Input: part model. Units: mm. Frame: model coordinates. Face numbers are marked on the shaded views. A direction names the side the tool comes from. Give positions to 0.01 mm unless a question says otherwise; leave off trailing zeros. Order: outer loops, then holes, each group sorted by start corner. A loop starts at its lowest first (then second) coordinate and runs counter-clockwise, first axis right, second up. Notation, with made-up numbers: (51, -10.75) - (102, -10.75) arc R28 cw to (102, 8.25) - close; hole circle Ø1 at (56, 80). An arc over 180 degrees is marked (long way). Answer in a Markdown table with one row per item. Add a question column.
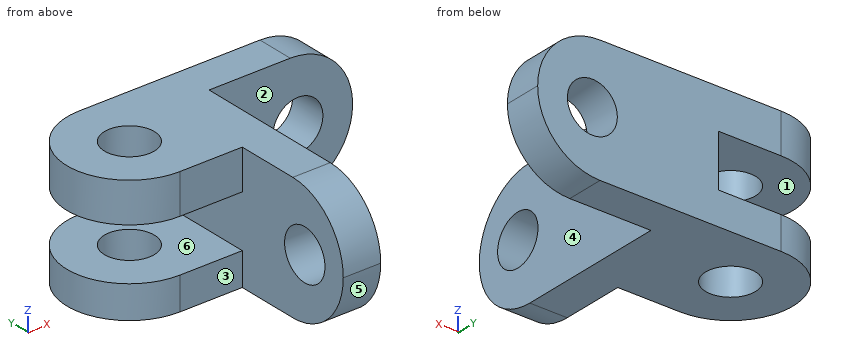
from build123d import *

# Parameters (mm, degrees)
SKETCH1_R               = 20
SKETCH1_R_2             = 8
BOSS_EXTRUDE1_DEPTH     = 20
FILLET1_R               = 20
SKETCH2_R               = 8
CUT_EXTRUDE2_DEPTH      = 16
SKETCH3_W               = 74.438735145
SKETCH3_H               = 16.753132604
CUT_EXTRUDE3_DEPTH      = 90.911067172
FILLET2_R               = 20
FILLET3_R               = 20
CUT_EXTRUDE4_DEPTH      = 82.877957962
CUT_EXTRUDE4_DEPTH_BACK = 82.877957962
SKETCH4_R               = 8


with BuildPart() as part:
    # Sketch1 → Boss-Extrude1 (new, symmetric)
    # profile 1 of 2: a face of its own
    with BuildSketch(Plane.XY):
        Circle(SKETCH1_R)
        Circle(SKETCH1_R_2, mode=Mode.SUBTRACT)
    # profile 2 of 2: a face of its own
    with BuildSketch(Plane.XY):
        with BuildLine():
            Line((78, 20), (0, 20))
            ThreePointArc((0, 20), (14.142135624, 14.142135624), (20, 0))
            ThreePointArc((20, 0), (14.142135624, -14.142135624), (0, -20))
            Line((0, -20), (20, -20))
            Line((20, -20), (20, -60))
            Line((20, -60), (32, -60))
            Line((32, -60), (32, 8))
            Line((32, 8), (78, 8))
            Line((78, 8), (78, 20))
        make_face()
    extrude(amount=BOSS_EXTRUDE1_DEPTH, both=True)

    # Fillet1
    fillet1_edges = [part.edges().sort_by_distance(p)[0] for p in [
        (78, 14, -20),
        (78, 14, 20),
    ]]
    fillet(fillet1_edges, radius=FILLET1_R - 0.0001)  # a hair under: the kernel refuses the full size

    # Sketch2 → Cut-Extrude2 (cut)
    with BuildSketch(Plane(origin=(0, 20, 0), x_dir=(1, 0, 0), z_dir=(0, 1, 0))):
        with Locations(Location((60.472902104, 0, 0), (0, 0, 180))):
            Circle(SKETCH2_R)
    extrude(amount=-CUT_EXTRUDE2_DEPTH, mode=Mode.SUBTRACT)

    # Sketch3 → Cut-Extrude3 (cut, through all)
    with BuildSketch(Plane.XZ.offset(20)):
        with Locations((-17.219367573, -1.130171644)):
            Rectangle(SKETCH3_W, SKETCH3_H)
    extrude(amount=-CUT_EXTRUDE3_DEPTH, mode=Mode.SUBTRACT)

    # Fillet2
    fillet2_edges = [part.edges().sort_by_distance(p)[0] for p in [
        (26, -60, 20),
    ]]
    fillet(fillet2_edges, radius=FILLET2_R)

    # Fillet3
    fillet3_edges = [part.edges().sort_by_distance(p)[0] for p in [
        (26, -60, -20),
    ]]
    fillet(fillet3_edges, radius=FILLET3_R - 0.0001)  # a hair under: the kernel refuses the full size

    # Sketch4 → Cut-Extrude4 (cut, two sides: drawn at the far end of the back side and taken through both)
    with BuildSketch(Plane(origin=(32, 0, 0), x_dir=(0, 0, -1), z_dir=(1, 0, 0)).offset(-CUT_EXTRUDE4_DEPTH_BACK)):
        with Locations(Location((0, -44.755854097, 0), (0, 0, 90))):
            Circle(SKETCH4_R)
    extrude(amount=CUT_EXTRUDE4_DEPTH + CUT_EXTRUDE4_DEPTH_BACK, mode=Mode.SUBTRACT)


solid = part.part
Q1. Line query: probe 1 along X at (y, z) = (0, -15); probe 2 along Y at (x, z) = (0, -14); probe 3 along Z at (x, y) = (-10, 10.5). Output: solid intervals per line, ascending.
Q2. Access query for the marked faces 1, 2 and 3. Directions: +Z, -Z, +X, -X, +Y, -Y. A direction counts if a zero-diameter tool reaches every point of the face in a straight line with its end or side. Return the directions, or none.
Q3. Section B-B, the plane z = 11.5. Return loops of the section in (x, y).
Q4. Pull-direction query (Z, two-part tool) for the marked faces 4, 5 and 6; classes: +Z half, -Z half, draft (parallel to the pull), parting line (faces both ways), or undercut.
Q5. Section C-C, the plane y = -42.5. Return loops of the section in (x, z), then the cut area to 3 significant figures.
Q6. Section D-D, the plane z = 4.5. Return loops of the section in (x, y), then the cut area to 3 significant figures.
Q7. Contact query for flat-ended pins moving along their axis: P1, Ø10, axis at x = 61.5, z = 15.5, coming from the -Y side; P2, Ø6.5, axis at x = 14.5, z = 12.5, coming from the -Y side; P3, Ø12, axis at x = -4.5, z = 3, coming from the +Y side. Output: stop coordinate, or through.
Q8. Section A-A, the plane y = 0. Return loops of the section in (x, z).
Computed:
| question | item | result |
|---|---|---|
| 1 | probe 1 | x = -20 to -8, 8 to 32 |
| 1 | probe 2 | y = -20 to -8, 8 to 20 |
| 1 | probe 3 | z = -20 to -9.51, 7.25 to 20 |
| 2 | face 1 | -X, +Y, -Y |
| 2 | face 2 | +Z, -Z, +X, -Y |
| 2 | face 3 | +Z, -Z, -X, -Y |
| 3 | outline | (0, -20) - (20, -20) - (20, -56.36) - (32, -56.36) - (32, 8) - (74.36, 8) - (74.36, 20) - (0, 20) arc R20 ccw to start; hole circle Ø16 at (0, 0) |
| 4 | face 4 | draft |
| 4 | face 5 | -Z half |
| 4 | face 6 | undercut |
| 5 | outline | (20, -19.84) - (32, -19.84) - (32, -7.68) - (20, -7.68) - close; (20, 7.68) - (32, 7.68) - (32, 19.84) - (20, 19.84) - close |
| 5 | area | 292 mm^2 |
| 6 | outline | (20, -59.49) - (32, -59.49) - (32, -51.37) - (20, -51.37) - close; (20, -38.14) - (32, -38.14) - (32, 8) - (53.86, 8) - (53.86, 20) - (20, 20) - close; (67.09, 8) - (77.49, 8) - (77.49, 20) - (67.09, 20) - close |
| 6 | area | 1,180 mm^2 |
| 7 | P1 | stops at y = 8 |
| 7 | P2 | stops at y = -20 |
| 7 | P3 | stops at y = 20 |
| 8 | outline | (-20, -20) - (-8, -20) - (-8, -9.51) - (-20, -9.51) - close; (-20, 7.25) - (-8, 7.25) - (-8, 20) - (-20, 20) - close; (8, -20) - (32, -20) - (32, 20) - (8, 20) - (8, 7.25) - (20, 7.25) - (20, -9.51) - (8, -9.51) - close |
